The model under review builds one solid part; all positions refer to its coordinate system, in mm. Face numbers are marked on the shaded views. A direction names the side the tool comes from. Coordinates: 2 decimals unless noted, no trailing zeros. Order: outer loops, then holes, each group sorted by start corner. A loop starts at its lowest first (then second) coordinate and runs counter-clockwise, first axis right, second up. Notation, with made-up numbers: M 86.5,33 L 123.5,33 A34 cw 123.5,69 Z; hole C 81.25,-3 d6. An arc over 180 degrees is marked long. One line per item, written item: value.
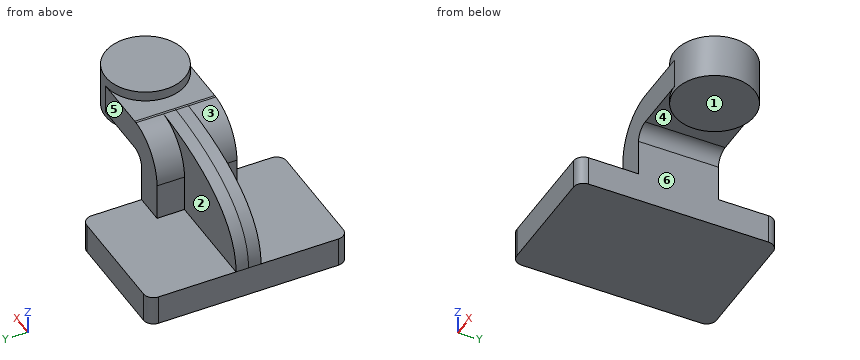
```python
from build123d import *

# Parameters (mm, degrees)
F1_DEPTH = 63.5
F0_W     = 25.4
F0_H     = 19.05
F2_DEPTH = 25.4
F3_DEPTH = 7.9375
F4_R     = 6.35


with BuildPart() as f1:
    # F0 (on Front) → F1 (new body, symmetric)
    with BuildSketch(Plane.XZ):
        Polygon((41.275, -9.525), (41.275, 9.525), (22.225, 9.525), (-41.275, 9.525), (-41.275, -9.525), align=None)
    extrude(amount=F1_DEPTH, both=True)

    # F0 (on Front) → F2 (join, symmetric)
    with BuildSketch(Plane.XZ):
        with BuildLine():
            Line((22.225, 9.525), (41.275, 9.525))
            Line((41.275, 9.525), (41.275, 33.02))
            ThreePointArc((41.275, 33.02), (43.6928335213, 38.8571664787), (49.53, 41.275))
            Line((49.53, 41.275), (60.325, 41.275))
            Line((60.325, 41.275), (60.325, 60.325))
            Line((60.325, 60.325), (49.53, 60.325))
            add(Edge.make_bspline(
                [(48.1194647713, 60.2885425971), (48.5932006273, 60.3022707881), (49.063439273, 60.3144056478), (49.53, 60.325)],
                knots=[102.663192175, 102.663192175, 102.663192175, 102.663192175, 104.0489693606, 104.0489693606, 104.0489693606, 104.0489693606], degree=3))
            ThreePointArc((48.1194647713, 60.2885425971), (29.730029174, 51.8222387042), (22.225, 33.02))
            Line((22.225, 33.02), (22.225, 9.525))
        make_face()
        with Locations((73.025, 50.8)):
            Rectangle(F0_W, F0_H)
    extrude(amount=F2_DEPTH, both=True)

    # F0 (on Front) → F3 (join, symmetric)
    with BuildSketch(Plane.XZ):
        with BuildLine():
            Line((-41.275, 9.525), (22.225, 9.525))
            Line((22.225, 9.525), (22.225, 33.02))
            ThreePointArc((22.225, 33.02), (29.730029174, 51.8222387042), (48.1194647713, 60.2885425971))
            add(Edge.make_bspline(
                [(-41.275, 9.525), (-41.2664891716, 49.5096992436), (13.0234654023, 59.2715104706), (48.1194647713, 60.2885425971)],
                knots=[0, 0, 0, 0, 102.663192175, 102.663192175, 102.663192175, 102.663192175], degree=3))
        make_face()
    extrude(amount=F3_DEPTH, both=True)

    # F4
    f4_edges = [f1.edges().sort_by_distance(p)[0] for p in [
        (41.275, -63.5, 0),
        (-41.275, -63.5, 0),
        (41.275, 63.5, 0),
        (-41.275, 63.5, 0),
    ]]
    fillet(f4_edges, radius=F4_R)

    # F0 (on Front) → F5 (revolve)
    with BuildSketch(Plane.XZ):
        Polygon((85.725, 60.325), (85.725, 41.275), (85.725, 38.1), (111.125, 38.1), (111.125, 66.675), (85.725, 66.675), align=None)
    revolve(axis=Axis((85.725, 0, 52.3875), (0, 0, 1)))


solid = f1.part
```
(1) We need section C-C, the plane x = 97.5. State the section outline as (y, z) points (3 decimals), plus the area to 3 significant figures.
Geometry results:
outline: M -22.506,38.1 L 22.506,38.1 L 22.506,66.675 L -22.506,66.675 Z
area: 1,290 mm2
(2) Insertion check: pin 1 Ø15 at (x, z) = (51, 46) entering from +Y; pin 2 Ø1 at (x, y) = (-19.5, -11.5) entering from +Z (3 decimals); pin 3 Ø5 at (y, z) = (14.5, 19.5) entering from -X (3 decimals). Each pin has a flat end and moves straight along its axis. Give the tip position at first contact, or say it passes through.
Geometry results:
pin 1: stops at y = 25.4
pin 2: stops at z = 9.525
pin 3: stops at x = 22.225
(3) We need section B-B, the plane y = -44. State the section outline as (x, z) points (3 decimals).
Geometry results:
outline: M -41.275,-9.525 L 41.275,-9.525 L 41.275,9.525 L -41.275,9.525 Z
(4) For L1, parallel to Y at x = 70, z = 43; L2, parallel to Z at x = 4, y = -21.5 (3 decimals); L3, parallel to X at y = 44.5, z = 4 (3 decimals), list the stretches that pass through material, from the lowest coordinate up.
Geometry results:
L1: y = -25.4 to 25.4
L2: z = -9.525 to 9.525
L3: x = -41.275 to 41.275
(5) Mouldability with a two-part tool opening along X and no side actions: class the marked faces 4, 5 and 6 as +X half, -X half, draft (parallel to the pull), parting line (faces both ways), or undercut.
Geometry results:
face 4: undercut
face 5: draft
face 6: +X half
(6) We need section A-A, the plane x = 70. State the section outline as (y, z) points (3 decimals).
Geometry results:
outline: M -25.4,41.275 L -19.947,41.275 L -19.947,38.1 L 19.947,38.1 L 19.947,41.275 L 25.4,41.275 L 25.4,60.325 L 19.947,60.325 L 19.947,66.675 L -19.947,66.675 L -19.947,60.325 L -25.4,60.325 Z
(7) Tool access review of the marked faces 1, 2 and 3: name each direction out of +Z, -Z, +X, -X, +Y, -Y from which nothing blocks a thin tool from reaching the whole face with its end or side.
Geometry results:
face 1: -Z, +X, +Y, -Y
face 2: +Z, -X, +Y
face 3: +Z, -X, -Y
